from build123d import *

# Parameters (mm, degrees)
F0_R     = 19
F0_R_2   = 16
F0_R_3   = 11
F1_DEPTH = 2
F2_DEPTH = 9
F3_R     = 1
F4_R     = 0.99999
F0_R_4   = 8
F5_DEPTH = 2


# Not quite as in the source:
# - a fillet or chamfer is up to 0.001 mm smaller than in the source, because OpenCascade refuses the exact size


with BuildPart() as f1:
    # F0 (on Top) → F1 (new body)
    with BuildSketch(Plane.XY):
        Circle(F0_R)
        Circle(F0_R_2, mode=Mode.SUBTRACT)
        Circle(F0_R_2)
        Circle(F0_R_3, mode=Mode.SUBTRACT)
    extrude(amount=F1_DEPTH)

    # F0 (on Top) → F2 (join)
    with BuildSketch(Plane.XY):
        Circle(F0_R_2)
        Circle(F0_R_3, mode=Mode.SUBTRACT)
    extrude(amount=F2_DEPTH)

    # F3
    f3_edges = [f1.edges().sort_by_distance(p)[0] for p in [
        (-19, 0, 2),
    ]]
    fillet(f3_edges, radius=F3_R)

    # F4 (radius 1 in the source; OpenCascade refuses exactly that, so slightly less here)
    f4_edges = [f1.edges().sort_by_distance(p)[0] for p in [
        (-19, 0, 0),
    ]]
    fillet(f4_edges, radius=F4_R)

    # F0 (on Top) → F5 (join)
    with BuildSketch(Plane.XY):
        Circle(F0_R_3)
        Circle(F0_R_4, mode=Mode.SUBTRACT)
    extrude(amount=F5_DEPTH)


solid = f1.part
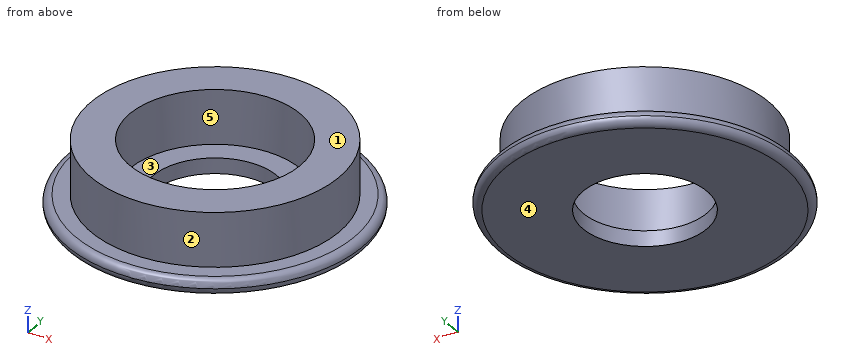
Design review of the part built by this model. Coordinates are the model's own, in mm. Face numbers are marked on the shaded views. A direction names the side the tool comes from. Coordinates: 2 decimals unless noted, no trailing zeros. Write each loop counter-clockwise with the first axis right and the second up, starting at its lowest first coordinate (ties: lowest second). Pieces come first, ordered by that corner, then holes. Notation, with made-up numbers: (-1, 65) -> (35, 65) arc R20 cw to (35, 73) -> close; hole circle Ø11 at (19.5, -28.75). An arc over 180 degrees is marked (long way). Write each question's results on one line, items separated by ' | '. Start each with the question number.
(1) Clearance check with flat-ended pins moving along their axes: P1, Ø13, axis at x = 0, y = 0, coming from the -Z side; P2, Ø2, axis at x = 12, z = 7, coming from the +Y side; P3, Ø11, axis at x = -4.5, y = -1.5, coming from the +Z side. State where each tip first meets the part, or that it passes through.
(2) For line 1 along Y through (x, z) = (0, 0.9); line 2 along Y through (x, z) = (0, 7.25); line 3 along Z through (x, y) = (10, -4.5), list the stretches that pass through material, from the lowest coordinate up. Write a range as from..to.
(3) Tool access review of the marked faces 4 and 5: name each direction out of +Z, -Z, +X, -X, +Y, -Y from which nothing blocks a thin tool from reaching the whole face with its end or side.
(4) The part is to be moulded in two halves that separate along Y. For the marked faces 1, 2 and 3, say which applies: pulls with the +Y half, pulls with the -Y half, needs draft (parallel to the pull), parting line crosses it, or undercut.
(5) Take a section at C-C on z = 4. Write out the cut boundary in (x, y), and give its area (3 significant figures).
Results found:
1) P1: passes through | P2: stops at y = 11.62 | P3: stops at z = 2
2) line 1: y = -18.99..-8, 8..18.99 | line 2: y = -16..-11, 11..16 | line 3: z = 0..2
3) face 4: -Z, +X, -X, +Y, -Y | face 5: +Z
4) face 1: needs draft | face 2: parting line crosses it | face 3: undercut
5) outline: circle Ø32 at (0, 0); hole circle Ø22 at (0, 0) | area: 424 mm2
